```python
from build123d import *

# Parameters (mm, degrees)
SKETCH1_W         = 68.58
SKETCH1_H         = 53.34
PCB_BASE_DEPTH    = 2.54
SKETCH1_4_W       = 73.66
SKETCH1_4_H       = 60.96
SKETCH1_4_W_2     = 68.58
SKETCH1_4_H_2     = 53.34
PCB_WALL_DEPTH    = 13.97
SKETCH3_R         = 1.651
BATTERY_GAP_DEPTH = 2.54


with BuildPart() as part:
    # Sketch1 → pcb-base (new body)
    with BuildSketch(Plane(origin=(0, 0, 0), x_dir=(1, 0, 0), z_dir=(0, 1, 0))):
        Rectangle(SKETCH1_W, SKETCH1_H)
    extrude(amount=PCB_BASE_DEPTH)

    # Sketch1<4> → pcb-wall (add)
    with BuildSketch(Plane(origin=(0, 0, 0), x_dir=(1, 0, 0), z_dir=(0, 1, 0))):
        Rectangle(SKETCH1_4_W, SKETCH1_4_H)
        Rectangle(SKETCH1_4_W_2, SKETCH1_4_H_2, mode=Mode.SUBTRACT)
    extrude(amount=PCB_WALL_DEPTH)

    # Sketch3 → battery-gap (cut)
    with BuildSketch(Plane.ZY.offset(36.83)):
        with Locations((20.32, 4.318)):
            Circle(SKETCH3_R)
    extrude(amount=-BATTERY_GAP_DEPTH, mode=Mode.SUBTRACT)


solid = part.part
```
Source: CAD feature listing. Evaluate the final solid. Frame: model axes, mm. A direction names the side the tool comes from. Coordinates: 2 decimals unless noted, no trailing zeros. Loops run counter-clockwise (first coordinate to the right, second up) from the corner with the lowest first, then second, coordinate; pieces in that order, holes last. Notation, with made-up numbers: (42, 66) - (92, 66) arc R26 cw to (92, 98) - close; hole circle Ø3 at (-29, 80.5). An arc over 180 degrees is marked (long way). Answer as CSV lines item,"result".
1. Contact query for a flat-ended pin moving along its axis: pin 1 (12 mm diameter, centred on x = 6, z = 3.5, fed in from +Y). Output: stop coordinate, or through.
Established:
pin 1,"stops at y = 2.54"
2. Mould query, pull axis X, two halves, no side actions, for faces 1 (the flat face through (34.29, 8, 0)), 2 (the flat face through (-3, 13.97, 27)), 3 (the flat face through (36.83, 7, 0)). Classes: released by +X, released by -X, zero draft, split by the parting line, or undercut.
Established:
face 1,"undercut"
face 2,"zero draft"
face 3,"released by +X"
3. Section D-D (z = -6). Return loops of the section in (x, y).
Established:
outline,"(-36.83, 0) - (36.83, 0) - (36.83, 13.97) - (34.29, 13.97) - (34.29, 2.54) - (-34.29, 2.54) - (-34.29, 13.97) - (-36.83, 13.97) - close"
4. Ray query, line 1 (X direction, y = 10.5, z = -20); line 2 (Y direction, x = -36, z = 20.32); line 3 (Z direction, x = 23, y = 9.5). Return the intervals inside material, ascending.
Established:
line 1,"x = -36.83 to -34.29, 34.29 to 36.83"
line 2,"y = 0 to 2.67, 5.97 to 13.97"
line 3,"z = -30.48 to -26.67, 26.67 to 30.48"
5. Section A-A (y = 7.75). Return loops of the section in (x, z).
Established:
outline,"(-36.83, -30.48) - (36.83, -30.48) - (36.83, 30.48) - (-36.83, 30.48) - close; hole (-34.29, -26.67) - (34.29, -26.67) - (34.29, 26.67) - (-34.29, 26.67) - close"
6. Reachability of faces 4 (the cylindrical face through (-35.578, 3.686, 21.845)), 5 (the flat face through (0, 8, 26.67)), 6 (the flat face through (-1, 7, -30.48)) from +Z, -Z, +X, -X, +Y, -Y: full face, straight path, thin tool, end or side. Return the list, or none.
Established:
face 4,"-X"
face 5,"+Y"
face 6,"-Z, +X, -X, +Y, -Y"
7. Section C-C (x = -27). Return loops of the section in (y, z).
Established:
outline,"(0, -30.48) - (13.97, -30.48) - (13.97, -26.67) - (2.54, -26.67) - (2.54, 26.67) - (13.97, 26.67) - (13.97, 30.48) - (0, 30.48) - close"
8. Section B-B (z = 20.32). Return loops of the section in (x, y), then the cut area to 3 significant figures.
Established:
outline,"(-36.83, 0) - (36.83, 0) - (36.83, 13.97) - (34.29, 13.97) - (34.29, 2.54) - (-34.29, 2.54) - (-34.29, 2.67) - (-36.83, 2.67) - close; (-36.83, 5.97) - (-34.29, 5.97) - (-34.29, 13.97) - (-36.83, 13.97) - close"
area,"237 mm2"
